Autodesk Inventor part; units mm, degrees
ref_plane "YZ Plane" through (0, 0, 0) normal (1, 0, 0) x (0, 1, 0)
ref_plane "XZ Plane" through (0, 0, 0) normal (0, 1, 0) x (-1, 0, 0)
ref_plane "XY Plane" through (0, 0, 0) normal (0, 0, 1) x (1, 0, 0)
sketch "Sketch1" plane through (0, 0, 0) normal (0, 0, 1) x (1, 0, 0)
  line L0 (-16, -12.5) -> (16, -12.5)
  line L1 (16, -12.5) -> (16, 12.5)
  line L2 (16, 12.5) -> (13, 12.5)
  line L3 (13, 12.5) -> (13, -9.5)
  line L4 (13, -9.5) -> (-13, -9.5)
  line L5 (-13, -9.5) -> (-13, 12.5)
  line L6 (-13, 12.5) -> (-16, 12.5)
  line L7 (-16, 12.5) -> (-16, -12.5)
  point P0 (0, 0)
  dimension "d0" = 32
  dimension "d1" = 25
  dimension "d2" = 3
  dimension "d3" = 90
  dimension "d4" = 22
  dimension "d5" = 26
  dimension "d6" = 22
  dimension "d7" = 3
  dimension "d8" = 25
  dimension "d10" = 12.5
  dimension "d11" = 16
extrude "Extrusion1" add sketch "Sketch1" against normal blind 203.2
chamfer "Chamfer1" distance 25 angle 30 1 edges at (14.5, 12.5, 0) measured on face at (4.3333, -11.5, 0)
chamfer "Chamfer2" distance 25 angle 30 1 edges at (14.5, 12.5, -203.2) measured on face at (4.3333, -11.5, -203.2)
equation "\"d5\" = d0 - 2 * d7"
properties part number "Chassis Corner"
Geometry: final body of the model. Coordinates: model frame, mm. A direction names the side the tool comes from. Coordinates: 2 decimals unless noted, no trailing zeros. Loops run counter-clockwise (first coordinate to the right, second up) from the corner with the lowest first, then second, coordinate; pieces in that order, holes last. Notation, with made-up numbers: (55, 30) -> (108, 30) arc R11 cw to (108, 47) -> close; hole circle Ø10 at (36.25, 42). An arc over 180 degrees is marked (long way). Use a Markdown table: item, result. Add a question column.
(1) Section query A-A, the plane y = 2. Return loops of the section in (x, z), plus the area to 3 significant figures.
(2) Access query for faces 1 (the flat face through (-13, 1, -100)), 2 (the flat face through (0, -12.5, -100)). Directions: +Z, -Z, +X, -X, +Y, -Y. A direction counts if a zero-diameter tool reaches every point of the face in a straight line with its end or side. Return the directions, or none.
(3) Line query: line 1 along X through (y, z) = (-6, -43.5); line 2 along Y through (x, z) = (-11, -109); line 3 along Z through (x, y) = (-1, -11). Output: solid intervals per line, ascending.
(4) Mould query, pull axis X, two halves, no side actions, for faces 3 (the flat face through (13, 2, -100)), 4 (the flat face through (16, 0, -100)), 5 (the flat face through (-1.26, -10.13, -201.83)). Classes: pulls with the +X half, pulls with the -X half, needs draft (parallel to the pull), parting line crosses it, or undercut.
(5) Section query C-C, the plane z = -184.5. Return loops of the section in (x, y), plus the area to 3 significant figures.
(6) Pin query (flat end, axial travel): pin 1 Ø5 at (x, z) = (7, -122) entering from +Y. Return the tip coordinate at first contact, or that it passes through.
(7) Section query D-D, the plane y = -6.25. Return loops of the section in (x, z).
Answer:
| question | item | result |
|---|---|---|
| 1 | outline | (-16, -194.83) -> (-13, -194.83) -> (-13, -8.37) -> (-16, -8.37) -> close; (13, -194.83) -> (16, -194.83) -> (16, -8.37) -> (13, -8.37) -> close |
| 1 | area | 1,120 mm^2 |
| 2 | face 1 | +Z, -Z, +Y |
| 2 | face 2 | +Z, -Z, +X, -X, -Y |
| 3 | line 1 | x = -16 to -13, 13 to 16 |
| 3 | line 2 | y = -12.5 to -9.5 |
| 3 | line 3 | z = -202.33 to -0.87 |
| 4 | face 3 | undercut |
| 4 | face 4 | pulls with the +X half |
| 4 | face 5 | needs draft |
| 5 | outline | (-16, -12.5) -> (16, -12.5) -> (16, 12.5) -> (13, 12.5) -> (13, -9.5) -> (-13, -9.5) -> (-13, 12.5) -> (-16, 12.5) -> close |
| 5 | area | 228 mm^2 |
| 6 | pin 1 | stops at y = -9.5 |
| 7 | outline | (-16, -199.59) -> (-13, -199.59) -> (-13, -3.61) -> (-16, -3.61) -> close; (13, -199.59) -> (16, -199.59) -> (16, -3.61) -> (13, -3.61) -> close |
